The model under review builds one solid part; all positions refer to its coordinate system, in mm. Face numbers are marked on the shaded views. A direction names the side the tool comes from. Coordinates: 2 decimals unless noted, no trailing zeros. Order: outer loops, then holes, each group sorted by start corner. A loop starts at its lowest first (then second) coordinate and runs counter-clockwise, first axis right, second up. Notation, with made-up numbers: M 18,61.5 L 55,61.5 A23 ccw 55,86.5 Z; hole C 27,10 d5. An arc over 180 degrees is marked long. One line per item, written item: value.
Autodesk Inventor part; units mm, degrees
ref_plane "YZ Plane" through (0, 0, 0) normal (1, 0, 0) x (0, 1, 0)
ref_plane "XZ Plane" through (0, 0, 0) normal (0, 1, 0) x (-1, 0, 0)
ref_plane "XY Plane" through (0, 0, 0) normal (0, 0, 1) x (1, 0, 0)
sketch "Эскиз1" plane through (0, 0, 0) normal (1, 0, 0) x (0, 1, 0)
  line L0 (-3.98, -3) -> (-3.38, 0)
  line L1 (-3.98, -3) -> (-56.02, -3)
  line L2 (-4.48, -22.93) -> (-4.48, -3)
  line L3 (-55.52, -22.93) -> (-55.52, -3)
  line L4 (-3.98, -3) -> (-56.02, -3)
  line L5 (-56.02, -3) -> (-56.62, 0)
  line L6 (-60, 0) -> (0, 0)
  line L7 (-60, 0) -> (-60, -22.93)
  line L8 (0, 0) -> (0, -22.93)
  line L9 (-60, -22.93) -> (0, -22.93)
  line L10 (-3.98, -3) -> (-3.98, -3)
  line L11 (-3.98, -3) -> (-3.38, 0)
  line L12 (-56.02, -3) -> (-56.02, -3)
  line L13 (-56.02, -3) -> (-56.62, 0)
  line L14 (-3.38, 0) -> (4.62, 0)
  line L15 (-56.62, 0) -> (-64.62, 0)
  line L16 (-64.62, 0) -> (-64.62, 3)
  line L17 (-64.62, 3) -> (4.62, 3)
  line L18 (4.62, 3) -> (4.62, 0)
  line L19 (-30, -3) -> (-51.25, -3)
  line L20 (-51.25, -3) -> (-8.75, -3)
  line L21 (-8.75, -3) -> (-8.75, -22.93)
  line L22 (-51.25, -3) -> (-51.25, -22.93)
  line L23 (-52.5, -22.93) -> (-51.25, -22.93)
  line L24 (-51.5625, -21.93) -> (-51.5625, -22.93)
  line L25 (-51.875, -21.93) -> (-51.25, -21.93)
  line L26 (-52.5, -22.93) -> (-51.25, -20.93)
  spline S0 degree 2 poles (-52.5, -22.93) (-51.1297, -22.7543) (-51.25, -20.93) knots 0 0 0 1 1 1
  line L27 (-8.75, -19) -> (-8.75, -12)
  line L28 (-8.75, -12) -> (-51.25, -12)
  line L29 (-30, 3) -> (-30, -22.93)
  line L30 (-8.75, -12) -> (-11.75, -12)
  line L31 (-30, -12) -> (-30, -14)
  line L32 (-11.75, -12) -> (-13.75, -14)
  line L33 (-11.75, -12) -> (-8.9216, -12) construction
  line L34 (-13.75, -14) -> (-30, -14)
  line L35 (2, 0) -> (0, 0)
  line L36 (-7.75, -4.6) -> (-8.75, -4.6)
  line L37 (-8.25, -4.6) -> (-8.25, -3)
  line L38 (-6.75, -3) -> (-8.75, -3)
  line L39 (-6.75, -3) -> (-8.75, -6.2)
  spline S1 degree 2 poles (-6.75, -3) (-8.9425, -3.2811) (-8.75, -6.2) knots 0 0 0 1 1 1
  spline S2 degree 2 poles (-53.25, -3) (-51.0575, -3.2811) (-51.25, -6.2) knots 0 0 0 1 1 1
  line L40 (-30, -14) -> (-25, -14)
  line L41 (-25, -14) -> (-27, -12)
  point P0 (-51.5625, -22.43)
  point P1 (-30, -15.93)
  point P2 (1.4531, 0)
  point P3 (-8.25, -3.8)
  point P4 (-51.75, -3.8)
  point P5 (-30, -3)
  point P6 (-53.25, -3)
  point P7 (-51.25, -5.3265)
  point P8 (-8.75, -5.3265)
  dimension "d0" = 0
  dimension "d1" = 0
  dimension "d2" = 8
  dimension "d3" = 8
  dimension "d4" = 3
  dimension "d5" = 21.25
  dimension "d6" = 42.5
  dimension "d11" = 7
  dimension "d13" = 3
  dimension "d14" = 2
  dimension "d15" = 135
  dimension "d20" = 0
  dimension "d21" = 0
  dimension "d22" = 9
  dimension "d23" = 5
revolve "Вращение1" add sketch "Эскиз1" angle 360 about axis through (0, -30, 3) along (0, 0, -1) contours L29 L1 L5 L6 | L6 L15 L16 L17 L29 | L1 L21 S1 L28 L29 | L22 S2 L1 | L28 L32 L34 L41
sketch "Эскиз4" plane through (0, -30, 3) normal (0, 0, 1) x (1, 0, 0)
  line L0 (-1.2721, 9.2093) -> (-2.8003, 12.1239)
  line L1 (-2.8003, 12.1239) -> (-1.0404, 14.9046)
  line L2 (-1.0404, 14.9046) -> (2.2478, 14.7708)
  line L3 (2.2478, 14.7708) -> (3.776, 11.8563)
  line L4 (3.776, 11.8563) -> (2.0161, 9.0755)
  line L5 (2.0161, 9.0755) -> (-1.2721, 9.2093)
  circle A0 centre (0.4878, 11.9901) radius 1.7
  line L6 (-11.8997, 3.6368) -> (-13.428, 6.5513)
  line L7 (-13.428, 6.5513) -> (-11.668, 9.3321)
  line L8 (-11.668, 9.3321) -> (-8.3798, 9.1983)
  line L9 (-8.3798, 9.1983) -> (-6.8516, 6.2837)
  line L10 (-6.8516, 6.2837) -> (-8.6116, 3.503)
  line L11 (-8.6116, 3.503) -> (-11.8997, 3.6368)
  line L12 (-9.0994, -8.4871) -> (-12.3876, -8.3533)
  line L13 (-12.3876, -8.3533) -> (-13.9158, -5.4388)
  line L14 (-13.9158, -5.4388) -> (-12.1559, -2.658)
  line L15 (-12.1559, -2.658) -> (-8.8677, -2.7918)
  line L16 (-8.8677, -2.7918) -> (-7.3395, -5.7063)
  line L17 (-7.3395, -5.7063) -> (-9.0994, -8.4871)
  line L18 (2.8003, -12.1239) -> (1.0404, -14.9046)
  line L19 (1.0404, -14.9046) -> (-2.2478, -14.7708)
  line L20 (-2.2478, -14.7708) -> (-3.776, -11.8563)
  line L21 (-3.776, -11.8563) -> (-2.0161, -9.0755)
  line L22 (-2.0161, -9.0755) -> (1.2721, -9.2093)
  line L23 (1.2721, -9.2093) -> (2.8003, -12.1239)
  line L24 (11.8997, -3.6368) -> (13.428, -6.5513)
  line L25 (13.428, -6.5513) -> (11.668, -9.3321)
  line L26 (11.668, -9.3321) -> (8.3798, -9.1983)
  line L27 (8.3798, -9.1983) -> (6.8516, -6.2837)
  line L28 (6.8516, -6.2837) -> (8.6116, -3.503)
  line L29 (8.6116, -3.503) -> (11.8997, -3.6368)
  line L30 (9.0994, 8.4871) -> (12.3876, 8.3533)
  line L31 (12.3876, 8.3533) -> (13.9158, 5.4388)
  line L32 (13.9158, 5.4388) -> (12.1559, 2.658)
  line L33 (12.1559, 2.658) -> (8.8677, 2.7918)
  line L34 (8.8677, 2.7918) -> (7.3395, 5.7063)
  line L35 (7.3395, 5.7063) -> (9.0994, 8.4871)
  point P0 (0, 30)
extrude "Выдавливание3" cut sketch "Эскиз4" against normal blind 10 contours L0 L1 L2 L3 L4 L5 | A0 | L6 L7 L8 L9 L10 L11 | L12 L13 L14 L15 L16 L17 | L18 L19 L20 L21 L22 L23 | L24 L25 L26 L27 L28 L29 | L30 L31 L32 L33 L34 L35
sketch "Эскиз5" plane through (0, -30, -7) normal (0, 0, 1) x (1, 0, 0)
  circle A0 centre (0.4878, 11.9901) radius 1.7
  circle A1 centre (10.6276, 5.5726) radius 1.7
  circle A2 centre (10.1398, -6.4175) radius 1.7
  circle A3 centre (-0.4878, -11.9901) radius 1.7
  circle A4 centre (-10.6276, -5.5726) radius 1.7
  circle A5 centre (-10.1398, 6.4175) radius 1.7
  point P0 (0, 30)
extrude "Выдавливание4" cut sketch "Эскиз5" against normal blind 10
sketch "Эскиз6" plane through (0, -30, 3) normal (0, 0, 1) x (1, 0, 0)
  circle A0 centre (0, 0) radius 3
  point P0 (0, 30)
  dimension "d28" = 6
extrude "Выдавливание5" cut sketch "Эскиз6" against normal blind 20
sketch "Эскиз7" plane through (0, -30, -14) normal (0, 0, -1) x (-1, 0, 0)
  line L0 (0, 0) -> (0, 4.2)
  line L1 (2.4249, 4.2) -> (4.8497, 0)
  line L2 (4.8497, 0) -> (2.4249, -4.2)
  line L3 (2.4249, -4.2) -> (-2.4249, -4.2)
  line L4 (-2.4249, -4.2) -> (-4.8497, 0)
  line L5 (-4.8497, 0) -> (-2.4249, 4.2)
  line L6 (-2.4249, 4.2) -> (2.4249, 4.2)
  point P0 (0, 30)
  dimension "d31" = 4.2
extrude "Выдавливание6" cut sketch "Эскиз7" against normal blind 8
properties part number "tire vtulka2"
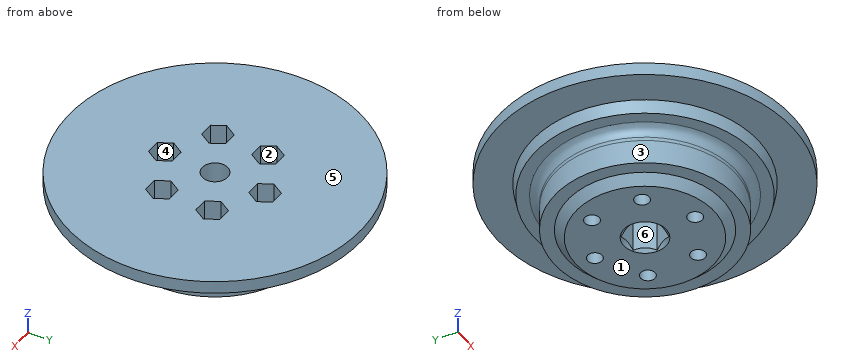
(1) We need section A-A, the plane z = -1.5. Count the separate pieces of the cut face and the enclosed holes in it, plus the area to 3 significant figures.
Geometry results:
separate pieces: 1
enclosed holes: 7
area: 1,980 mm2
(2) Tool access review of the marked faces 4, 5 and 6: name each direction out of +Z, -Z, +X, -X, +Y, -Y from which nothing blocks a thin tool from reaching the whole face with its end or side.
Geometry results:
face 4: +Z
face 5: +Z, +X, -X, +Y, -Y
face 6: -Z
(3) Mouldability with a two-part tool opening along X and no side actions: class the marked faces 1, 2 and 3 as +X half, -X half, draft (parallel to the pull), parting line (faces both ways), or undercut.
Geometry results:
face 1: draft
face 2: undercut
face 3: parting line
(4) We need section C-C, the plane x = 29. State the section outline as (y, z) points, plus the area to 3 significant figures.
Geometry results:
outline: M -48.91,0 L -11.09,0 L -11.09,3 L -48.91,3 Z
area: 113 mm2
(5) Insertion check: pin 1 Ø8 at (x, y) = (-23, -32.5) entering from -Z; pin 2 Ø3 at (x, y) = (10.14, -36.42) entering from +Z; pin 3 Ø1.7 at (x, y) = (2, -17.5) entering from +Z; pin 4 Ø3 at (x, y) = (-23.5, -4) entering from -Z. Each pin has a flat end and moves straight along its axis. Give the tip position at first contact, or say it passes through.
Geometry results:
pin 1: stops at z = -12
pin 2: passes through
pin 3: stops at z = -7
pin 4: stops at z = 0
(6) For L1, parallel to Y at x = -9, z = -5.25; L2, parallel to Y at x = -8, z = -5.75; L3, parallel to Y at x = 0, z = -3.5, list the stretches that pass through material, from the lowest coordinate up.
Geometry results:
L1: y = -49.26 to -38.33, -32.79 to -26.48, -20.78 to -10.74
L2: y = -49.67 to -36.75, -34.45 to -25.53, -21.53 to -10.33
L3: y = -52.03 to -44.86, -39.16 to -33, -27 to -20.84, -15.14 to -7.97
